from build123d import *

# Parameters (mm, degrees)
BOSS_EXTRUDE2_DEPTH = 4
SKETCH24_W          = 3
SKETCH24_H          = 8
BOSS_EXTRUDE3_DEPTH = 25.13
SKETCH25_R          = 1.75
SKETCH25_R_2        = 1.750000009
CUT_EXTRUDE1_DEPTH  = 4
SKETCH26_W          = 40.2
SKETCH26_H          = 4
BOSS_EXTRUDE4_DEPTH = 0.65
SKETCH27_R          = 1.25
CUT_EXTRUDE2_DEPTH  = 5


with BuildPart() as part:
    # Sketch23 → Boss-Extrude2 (new body)
    with BuildSketch(Plane(origin=(0, 0, 0), x_dir=(1, 0, 0), z_dir=(0, 1, 0))):
        Polygon((-77.074690926, 0), (-63.824690926, 0), (-63.824690926, -8), (-60.824690926, -8), (-60.824690926, 0), (-34.374690926, 0), (-34.374690926, 40.2), (-60.824690926, 40.2), (-60.824690926, 48.2), (-63.824690926, 48.2), (-63.824690926, 40.2), (-77.074690926, 40.2), align=None)
    extrude(amount=BOSS_EXTRUDE2_DEPTH)

    # Sketch24 → Boss-Extrude3 (add)
    with BuildSketch(Plane(origin=(0, 4, 0), x_dir=(1, 0, 0), z_dir=(0, 1, 0))):
        with Locations((-62.324690926, -4)):
            Rectangle(SKETCH24_W, SKETCH24_H)
        with Locations((-62.324690926, 44.2)):
            Rectangle(SKETCH24_W, SKETCH24_H)
    extrude(amount=BOSS_EXTRUDE3_DEPTH)

    # Sketch25 → Cut-Extrude1 (cut)
    with BuildSketch(Plane.ZY.offset(63.824690926)):
        with Locations((4.799999987, 9.375)):
            Circle(SKETCH25_R)
        with Locations((-45, 9.375)):
            Circle(SKETCH25_R)
        with Locations((-45, 19.725)):
            Circle(SKETCH25_R)
        with Locations((4.799999987, 19.725)):
            Circle(SKETCH25_R_2)
    extrude(amount=-CUT_EXTRUDE1_DEPTH, mode=Mode.SUBTRACT)

    # Sketch26 → Boss-Extrude4 (add)
    with BuildSketch(Plane(origin=(-34.374690926, 0, 0), x_dir=(0, 0, -1), z_dir=(1, 0, 0))):
        with Locations((20.1, 2)):
            Rectangle(SKETCH26_W, SKETCH26_H)
    extrude(amount=BOSS_EXTRUDE4_DEPTH)

    # Sketch27 → Cut-Extrude2 (cut)
    with BuildSketch(Plane(origin=(0, 4, 0), x_dir=(1, 0, 0), z_dir=(0, 1, 0))):
        with Locations(Location((-36.724690926, 32.192020694, 0), (0, 0, 270))):
            Circle(SKETCH27_R)
        with Locations(Location((-36.724690926, 24.2, 0), (0, 0, 270))):
            Circle(SKETCH27_R)
        with Locations(Location((-36.724690926, 16.2, 0), (0, 0, 270))):
            Circle(SKETCH27_R)
        with Locations(Location((-36.724690926, 8.2, 0), (0, 0, 270))):
            Circle(SKETCH27_R)
    extrude(amount=-CUT_EXTRUDE2_DEPTH, mode=Mode.SUBTRACT)


solid = part.part
Source: CAD feature listing. Evaluate the final solid. Frame: model axes, mm. A direction names the side the tool comes from. Coordinates: 2 decimals unless noted, no trailing zeros. Order: outer loops, then holes, each group sorted by start corner. A loop starts at its lowest first (then second) coordinate and runs counter-clockwise, first axis right, second up. Notation, with made-up numbers: M -4.75,70.25 L 26.25,70.25 A15 ccw 26.25,97.25 Z; hole C 71,84 d11. An arc over 180 degrees is marked long. Write each question's results on one line, items separated by ' | '. Start each with the question number.
Item 1: Line query: probe 1 along X at (y, z) = (2.7, -24.2); probe 2 along Y at (x, z) = (-49.5, -34); probe 3 along X at (y, z) = (25.25, 5.5). Output: solid intervals per line, ascending.
Item 2: Cut plane C-C (z = -24.2). Return loops of the section in (x, y).
Item 3: First-contact query: pin 1 Ø8 at (y, z) = (10.5, -42) entering from +X; pin 2 Ø1.2 at (x, y) = (-49, 2) entering from +Z; pin 3 Ø3 at (x, y) = (-43.5, 3) entering from -Z; pin 4 Ø1.5 at (x, z) = (-36.72, -16.2) entering from +Y (3 decimals). Flat tips, straight axial feed; report the tip coordinate or a pass-through.
Item 4: Cut plane B-B (y = 27.25). Return loops of the section in (x, z), and give its area (3 significant figures).
Item 5: Cut plane D-D (y = 19). Return loops of the section in (x, z).
Item 6: Cut plane A-A (z = 4.8). Return loops of the section in (x, y) (3 decimals).
Item 7: Set-up query: faces 1 (the face through (-70, 2, -40.2)), 2 (the face through (-47, 2, -40.2)), 3 (the face through (-62, 16, 0)). Return all of +Z, -Z, +X, -X, +Y, -Y with unobstructed straight access to the full face (end or side cutting, diameter ignored); none if empty.
Item 8: Draft query along X for faces 4 (the face through (-60.825, 14, -44)), 5 (the face through (-62.35, 20.91, 3.51)), 6 (the face through (-35.485, 2.028, -8.363)). Return one class per face: pulls with the +X half, pulls with the -X half, needs draft (parallel to the pull), parting line crosses it, or undercut.
Checked values:
1) probe 1: x = -77.07 to -37.97, -35.47 to -33.72 | probe 2: y = 0 to 4 | probe 3: x = -63.82 to -60.82
2) outline: M -77.07,0 L -37.97,0 L -37.97,4 L -77.07,4 Z; M -35.47,0 L -33.72,0 L -33.72,4 L -35.47,4 Z
3) pin 1: stops at x = -60.82 | pin 2: stops at z = 0 | pin 3: stops at z = -40.2 | pin 4: passes through
4) outline: M -63.82,-48.2 L -60.82,-48.2 L -60.82,-40.2 L -63.82,-40.2 Z; M -63.82,0 L -60.82,0 L -60.82,8 L -63.82,8 Z | area: 48.0 mm2
5) outline: M -63.82,-48.2 L -60.82,-48.2 L -60.82,-46.59 L -63.82,-46.59 Z; M -63.82,-43.41 L -60.82,-43.41 L -60.82,-40.2 L -63.82,-40.2 Z; M -63.82,0 L -60.82,0 L -60.82,3.21 L -63.82,3.21 Z; M -63.82,6.39 L -60.82,6.39 L -60.82,8 L -63.82,8 Z
6) outline: M -63.825,0 L -60.825,0 L -60.825,7.625 L -63.825,7.625 Z; M -63.825,11.125 L -60.825,11.125 L -60.825,17.975 L -63.825,17.975 Z; M -63.825,21.475 L -60.825,21.475 L -60.825,29.13 L -63.825,29.13 Z
7) face 1: -Z, -X, +Y, -Y | face 2: -Z, +X, +Y, -Y | face 3: +X, -X, +Y
8) face 4: pulls with the +X half | face 5: needs draft | face 6: undercut
